Read the model definition and answer for the solid it produces. Units are mm, in the model's axes. Face numbers are marked on the shaded views. A direction names the side the tool comes from. Round coordinates to 2 decimals unless told otherwise and drop trailing zeros. Answer as CSV lines item,"result".
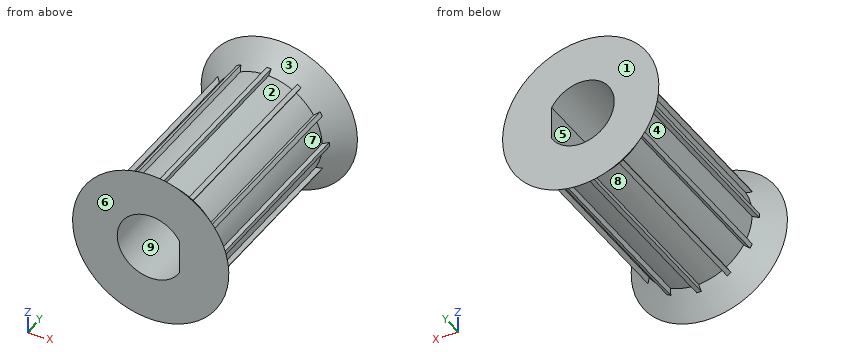
```python
from build123d import *

# Parameters (mm, degrees)
F1_DEPTH = 10


with BuildPart() as f1:
    # F0 (on Front) → F1 (new body)
    with BuildSketch(Plane.XZ):
        with BuildLine():
            ThreePointArc((-0.1, 2.497999), (0, 2.5), (0.1, 2.497999))
            Line((0.1, 2.497999), (0.1, 2.7))
            Line((0.1, 2.7), (-0.1, 2.7))
            Line((-0.1, 2.7), (-0.1, 2.497999))
        make_face()
        with BuildLine():
            ThreePointArc((-1.335602, 2.113331), (-1.25, 2.165064), (-1.162397, 2.213331))
            Line((-1.162397, 2.213331), (-1.263397, 2.388269))
            Line((-1.263397, 2.388269), (-1.436603, 2.288269))
            Line((-1.436603, 2.288269), (-1.335602, 2.113331))
        make_face()
        with BuildLine():
            ThreePointArc((-2.213331, 1.162397), (-2.165064, 1.25), (-2.113331, 1.335602))
            Line((-2.113331, 1.335602), (-2.288269, 1.436603))
            Line((-2.288269, 1.436603), (-2.388269, 1.263397))
            Line((-2.388269, 1.263397), (-2.213331, 1.162397))
        make_face()
        with BuildLine():
            ThreePointArc((-2.497999, -0.1), (-2.5, 0), (-2.497999, 0.1))
            Line((-2.497999, 0.1), (-2.7, 0.1))
            Line((-2.7, 0.1), (-2.7, -0.1))
            Line((-2.7, -0.1), (-2.497999, -0.1))
        make_face()
        with BuildLine():
            Line((-2.288269, -1.436603), (-2.113331, -1.335602))
            ThreePointArc((-2.113331, -1.335602), (-2.165064, -1.25), (-2.213331, -1.162397))
            Line((-2.213331, -1.162397), (-2.388269, -1.263397))
            Line((-2.388269, -1.263397), (-2.288269, -1.436603))
        make_face()
        with BuildLine():
            Line((-1.263397, -2.388269), (-1.162397, -2.213331))
            ThreePointArc((-1.162397, -2.213331), (-1.25, -2.165064), (-1.335602, -2.113331))
            Line((-1.335602, -2.113331), (-1.436603, -2.288269))
            Line((-1.436603, -2.288269), (-1.263397, -2.388269))
        make_face()
        with BuildLine():
            Line((0.1, -2.7), (0.1, -2.497999))
            ThreePointArc((0.1, -2.497999), (0, -2.5), (-0.1, -2.497999))
            Line((-0.1, -2.497999), (-0.1, -2.7))
            Line((-0.1, -2.7), (0.1, -2.7))
        make_face()
        with BuildLine():
            Line((1.436603, -2.288269), (1.335602, -2.113331))
            ThreePointArc((1.335602, -2.113331), (1.25, -2.165064), (1.162397, -2.213331))
            Line((1.162397, -2.213331), (1.263397, -2.388269))
            Line((1.263397, -2.388269), (1.436603, -2.288269))
        make_face()
        with BuildLine():
            Line((2.388269, -1.263397), (2.213331, -1.162397))
            ThreePointArc((2.213331, -1.162397), (2.165064, -1.25), (2.113331, -1.335602))
            Line((2.113331, -1.335602), (2.288269, -1.436603))
            Line((2.288269, -1.436603), (2.388269, -1.263397))
        make_face()
        with BuildLine():
            ThreePointArc((2.497999, 0.1), (2.4995, 0.05001), (2.5, 0))
            ThreePointArc((2.5, 0), (2.4995, -0.05001), (2.497999, -0.1))
            Line((2.497999, -0.1), (2.7, -0.1))
            Line((2.7, -0.1), (2.7, 0.1))
            Line((2.7, 0.1), (2.497999, 0.1))
        make_face()
        with BuildLine():
            ThreePointArc((2.113331, 1.335602), (2.165064, 1.25), (2.213331, 1.162397))
            Line((2.213331, 1.162397), (2.388269, 1.263397))
            Line((2.388269, 1.263397), (2.288269, 1.436603))
            Line((2.288269, 1.436603), (2.113331, 1.335602))
        make_face()
        with BuildLine():
            ThreePointArc((1.162397, 2.213331), (1.25, 2.165064), (1.335602, 2.113331))
            Line((1.335602, 2.113331), (1.436603, 2.288269))
            Line((1.436603, 2.288269), (1.263397, 2.388269))
            Line((1.263397, 2.388269), (1.162397, 2.213331))
        make_face()
        with BuildLine():
            ThreePointArc((2.497999, -0.1), (2.4995, -0.05001), (2.5, 0))
            ThreePointArc((2.5, 0), (2.4995, 0.05001), (2.497999, 0.1))
            ThreePointArc((2.497999, 0.1), (2.414815, 0.647048), (2.213331, 1.162397))
            ThreePointArc((2.213331, 1.162397), (2.165064, 1.25), (2.113331, 1.335602))
            ThreePointArc((2.113331, 1.335602), (1.767767, 1.767767), (1.335602, 2.113331))
            ThreePointArc((1.335602, 2.113331), (1.25, 2.165064), (1.162397, 2.213331))
            ThreePointArc((1.162397, 2.213331), (0.647048, 2.414815), (0.1, 2.497999))
            ThreePointArc((0.1, 2.497999), (0, 2.5), (-0.1, 2.497999))
            ThreePointArc((-0.1, 2.497999), (-0.647048, 2.414815), (-1.162397, 2.213331))
            ThreePointArc((-1.162397, 2.213331), (-1.25, 2.165064), (-1.335602, 2.113331))
            ThreePointArc((-1.335602, 2.113331), (-1.767767, 1.767767), (-2.113331, 1.335602))
            ThreePointArc((-2.113331, 1.335602), (-2.165064, 1.25), (-2.213331, 1.162397))
            ThreePointArc((-2.213331, 1.162397), (-2.414815, 0.647048), (-2.497999, 0.1))
            ThreePointArc((-2.497999, 0.1), (-2.5, 0), (-2.497999, -0.1))
            ThreePointArc((-2.497999, -0.1), (-2.414815, -0.647048), (-2.213331, -1.162397))
            ThreePointArc((-2.213331, -1.162397), (-2.165064, -1.25), (-2.113331, -1.335602))
            ThreePointArc((-2.113331, -1.335602), (-1.767767, -1.767767), (-1.335602, -2.113331))
            ThreePointArc((-1.335602, -2.113331), (-1.25, -2.165064), (-1.162397, -2.213331))
            ThreePointArc((-1.162397, -2.213331), (-0.647048, -2.414815), (-0.1, -2.497999))
            ThreePointArc((-0.1, -2.497999), (0, -2.5), (0.1, -2.497999))
            ThreePointArc((0.1, -2.497999), (0.647048, -2.414815), (1.162397, -2.213331))
            ThreePointArc((1.162397, -2.213331), (1.25, -2.165064), (1.335602, -2.113331))
            ThreePointArc((1.335602, -2.113331), (1.767767, -1.767767), (2.113331, -1.335602))
            ThreePointArc((2.113331, -1.335602), (2.165064, -1.25), (2.213331, -1.162397))
            ThreePointArc((2.213331, -1.162397), (2.414815, -0.647048), (2.497999, -0.1))
        make_face()
        with BuildLine():
            ThreePointArc((1.3, -0.748331), (-1.5, 0), (1.3, 0.748331))
            Line((1.3, 0.748331), (1.3, -0.748331))
        make_face(mode=Mode.SUBTRACT)
    extrude(amount=F1_DEPTH)

    # F2 (on Right) → F3 (revolve)
    with BuildSketch(Plane.YZ):
        Polygon((-9, 2.5), (-10, 3.5), (-10, 2.5), align=None)
        Polygon((-1, 2.5), (0, 2.5), (0, 3.5), align=None)
    revolve(axis=Axis((0, -5.253473, 0), (0, 1, 0)))


solid = f1.part
```
1) Determine the mould class of the marked faces 6, 7, 8 and 9 for opening direction X: released by +X, released by -X, zero draft, split by the parting line, or undercut.
Evaluation:
face 6,"zero draft"
face 7,"released by +X"
face 8,"undercut"
face 9,"undercut"
2) A tool of negligible diameter and unlimited length cuts with its end or side. For the marked faces 1, 2, 3, 4 and 5, from which of +Z, -Z, +X, -X, +Y, -Y can it reach the whole face along a straight path? Write none if from no direction.
Evaluation:
face 1,"+Z, -Z, +X, -X, +Y"
face 2,"+Z"
face 3,"none"
face 4,"-X"
face 5,"+Y, -Y"
3) Straight lines are drawn through the part: line 1 (Z direction, x = 0, y = -3); line 2 (X direction, y = -4.75, z = 0); line 3 (Y direction, x = 3, z = 0). For each, find the intervals that lie inside material, in ascending order.
Evaluation:
line 1,"z = -2.7 to -1.5, 1.5 to 2.7"
line 2,"x = -2.7 to -1.5, 1.3 to 2.7"
line 3,"y = -10 to -9.5, -0.5 to 0"
4) Each of these flat-tipped pins is pushed along its axis until it touches: P1, Ø3, axis at y = -3, z = -2.5, coming from the +X side; P2, Ø1.6, axis at y = -3, z = 0.5, coming from the -X side; P3, Ø1.5, axis at x = -1, y = -7.5, coming from the -Z side. Where does it stop, or does it pass through?
Evaluation:
P1,"stops at x = 2.39"
P2,"stops at x = -2.7"
P3,"stops at z = -2.49"
